```python
from build123d import *

# Parameters (mm, degrees)
F0_W           = 38.1
F0_H           = 25.4
F0_R           = 6.35
F1_DEPTH       = 44.45
F2_W           = 88.9
F2_H           = 6.35
F3_DEPTH       = 19.05
F5_D           = 8.73125
F5_DEPTH       = 19.05
F5_TIP         = 2.6231321399
F7_D           = 3.175
F7_DEPTH       = 12.7
F7_CBORE_D     = 4.7752
F7_CBORE_DEPTH = 3.175
F7_TIP         = 0.9538662327
F9_D           = 3.556


with BuildPart() as f1:
    # F0 (on Right) → F1 (new body, symmetric)
    with BuildSketch(Plane.YZ):
        Rectangle(F0_W, F0_H)
        Circle(F0_R, mode=Mode.SUBTRACT)
    extrude(amount=F1_DEPTH, both=True)

    # F2 (on face) → F3 (cut)
    with BuildSketch(Plane.XY.offset(12.7)):
        with BuildLine():
            Line((-9.525, 19.05), (-44.45, 19.05))
            Line((-44.45, 19.05), (-44.45, 12.7))
            Line((-44.45, 12.7), (-15.875, 12.7))
            ThreePointArc((-15.875, 12.7), (-11.3848719395, 14.5598719395), (-9.525, 19.05))
        make_face()
        with BuildLine():
            Line((44.45, 12.7), (44.45, 19.05))
            Line((44.45, 19.05), (9.525, 19.05))
            ThreePointArc((9.525, 19.05), (11.3848719395, 14.5598719395), (15.875, 12.7))
            Line((15.875, 12.7), (44.45, 12.7))
        make_face()
        with Locations((0, -15.875)):
            Rectangle(F2_W, F2_H)
    extrude(amount=-F3_DEPTH, mode=Mode.SUBTRACT)

    # F5
    with Locations(Plane(origin=(0, 19.05, 0), x_dir=(-1, 0, 0), z_dir=(0, 1, 0))):
        with Locations((0, 0)):
            Hole(F5_D / 2, depth=F5_DEPTH)
            with Locations((0, 0, -(F5_DEPTH + F5_TIP / 2))):  # 118° drill point
                Cone(0, F5_D / 2, F5_TIP, mode=Mode.SUBTRACT)

    # F7
    with Locations(Plane.XZ.offset(12.7)):
        with Locations((-31.75, 0), (31.75, 0)):
            CounterBoreHole(F7_D / 2, F7_CBORE_D / 2, F7_CBORE_DEPTH, depth=F7_DEPTH)
            with Locations((0, 0, -(F7_DEPTH + F7_TIP / 2))):  # 118° drill point
                Cone(0, F7_D / 2, F7_TIP, mode=Mode.SUBTRACT)

    # F9 (through all)
    with Locations(Plane.XY.offset(-6.35)):
        with Locations((-41.275, 15.875), (-15.875, 15.875), (15.875, 15.875), (41.275, 15.875), (41.275, -15.875), (15.875, -15.875), (-15.875, -15.875), (-41.275, -15.875)):
            Hole(F9_D / 2)


solid = f1.part
```
CAD build for the part. Positions are in the model's coordinates, mm. A direction names the side the tool comes from. Give positions to 0.01 mm unless a question says otherwise; leave off trailing zeros. Write each loop counter-clockwise with the first axis right and the second up, starting at its lowest first coordinate (ties: lowest second). Pieces come first, ordered by that corner, then holes. Notation, with made-up numbers: (25, 6) -> (83, 6) arc R10 ccw to (83, 21) -> close; hole circle Ø10 at (0, 15.5). An arc over 180 degrees is marked (long way). Write each question's results on one line, items separated by ' | '.
1. Which spindle directions (+Z, -Z, +X, -X, +Y, -Y) get a long thin tool onto all of the face, cutting with end or side? Do faces 5 (the cylindrical face through (-11.435, 14.511, 3.308)), 6 (the flat face through (-1, -12.7, 3)), 7 (the flat face through (-30, -9.525, 0)), 8 (the cylindrical face through (4.033, 11.73, -1.672)), 9 (the flat face through (27, 16, -6.35)). Say none if no direction does.
Geometry check:
face 5: +Z, -X, +Y | face 6: +Z, +X, -X, -Y | face 7: -Y | face 8: +Y | face 9: +Z, +X, +Y
2. Cut at D-D, the plane y = -15. Write the cut outline in (x, z).
Geometry check:
outline: (-44.45, -12.7) -> (-42.82, -12.7) -> (-42.82, -6.35) -> (-44.45, -6.35) -> close; (-39.73, -12.7) -> (-17.42, -12.7) -> (-17.42, -6.35) -> (-39.73, -6.35) -> close; (-14.33, -12.7) -> (14.33, -12.7) -> (14.33, -6.35) -> (-14.33, -6.35) -> close; (17.42, -12.7) -> (39.73, -12.7) -> (39.73, -6.35) -> (17.42, -6.35) -> close; (42.82, -12.7) -> (44.45, -12.7) -> (44.45, -6.35) -> (42.82, -6.35) -> close
3. Wall check: probe 1 along X at (y, z) = (-6.9, 0); probe 2 along Z at (x, y) = (31.75, -7.65); probe 3 along X at (y, z) = (-11, -1). Give the ranges that are in metal, low to high. Write a range as [from, to].
Geometry check:
probe 1: [-44.45, -33.34], [-30.16, 30.16], [33.34, 44.45] | probe 2: [-12.7, -1.59], [1.59, 12.7] | probe 3: [-44.45, -33.92], [-29.58, 29.58], [33.92, 44.45]
4. Cut at A-A, the plane x = -25.5. Write the cut outline in (y, z).
Geometry check:
outline: (-19.05, -12.7) -> (19.05, -12.7) -> (19.05, -6.35) -> (12.7, -6.35) -> (12.7, 12.7) -> (-12.7, 12.7) -> (-12.7, -6.35) -> (-19.05, -6.35) -> close; hole circle Ø12.7 at (0, 0)
5. Cut at B-B, the plane y = -1. Write the cut outline in (x, z).
Geometry check:
outline: (-44.45, -12.7) -> (44.45, -12.7) -> (44.45, -6.27) -> (-44.45, -6.27) -> close; (-44.45, 6.27) -> (44.45, 6.27) -> (44.45, 12.7) -> (-44.45, 12.7) -> close
6. Drop flat-ended pins along their axis: P1, Ø3, axis at x = -41.275, y = -15.875, coming from the -Z side; P2, Ø10, axis at y = -0.5, z = -2.5, coming from the -X side; P3, Ø10, axis at x = 12.5, z = 1, coming from the -Y side; P4, Ø1.4, axis at x = 33, z = -1, coming from the -Y side (3 decimals). Give the stop position or say it passes through.
Geometry check:
P1: through | P2: x = -44.45 | P3: y = -12.7 | P4: y = -9.525
7. Two-plate mould, pull along Z, no slides. Class faces 1 (the flat face through (30, 12.7, 3)), 2 (the cylindrical face through (-30.164, -7.813, 0.07)), 3 (the cylindrical face through (-34.135, -11.135, 0.105)), 4 (the flat face through (-27, 16, -6.35)): pulls with the +Z half, pulls with the -Z half, needs draft (parallel to the pull), parting line crosses it, or undercut.
Geometry check:
face 1: needs draft | face 2: undercut | face 3: undercut | face 4: pulls with the +Z half
